Autodesk Inventor part; units mm, degrees
ref_plane "YZ Plane" through (0, 0, 0) normal (1, 0, 0) x (0, 1, 0)
ref_plane "XZ Plane" through (0, 0, 0) normal (0, 1, 0) x (-1, 0, 0)
ref_plane "XY Plane" through (0, 0, 0) normal (0, 0, 1) x (1, 0, 0)
sketch "Sketch1" plane through (0, 0, 0) normal (0, 0, 1) x (1, 0, 0)
  line L0 (0, 0) -> (20, 0)
  line L1 (20, 0) -> (20, 20)
  line L2 (15, 25) -> (5, 25)
  line L3 (0, 20) -> (0, 0)
  circle A0 centre (5, 12.5) radius 1.6
  circle A1 centre (15, 12.5) radius 1.6
  line L4 (5, 25) -> (0, 20)
  line L5 (15, 25) -> (20, 20)
  line L6 (2.1625, 0) -> (2.1625, -6.35)
  line L7 (2.1625, -6.35) -> (5.3375, -6.35)
  line L8 (5.3375, -6.35) -> (5.3375, 0)
  line L9 (14.6625, 0) -> (14.6625, -6.35)
  line L10 (14.6625, -6.35) -> (17.8375, -6.35)
  line L11 (17.8375, -6.35) -> (17.8375, 0)
  point P0 (20, 25)
  point P1 (0, 25)
  dimension "d0" = 25
  dimension "d1" = 20
  dimension "d2" = 3.2
  dimension "d3" = 5
  dimension "d4" = 12.5
  dimension "d7" = 5
  dimension "d8" = 12.5
  dimension "d9" = 5
  dimension "d10" = 5
  dimension "d11" = 5
  dimension "d12" = 5
  dimension "d13" = 3.175
  dimension "d14" = 6.35
  dimension "d15" = 9.325
  dimension "d16" = 2.1625
  dimension "d17" = 2.1625
extrude "Extrusion1" add sketch "Sketch1" along normal blind 3.175
sketch "Sketch2" plane through (14.6625, -6.35, 0) normal (0, -1, 0) x (1, 0, 0)
  line L0 (0, 0) -> (3.175, 0)
  line L1 (3.175, 0) -> (3.175, 3.175)
  line L2 (0, 3.175) -> (3.175, 3.175)
  line L3 (0, 0) -> (0, 3.175)
  circle A0 centre (1.5875, 1.5875) radius 1.5875
  point P0 (-14.6625, 0)
extrude "Extrusion2" cut sketch "Sketch2" against normal blind 6.35 contours L3 A0 L0 | A0 L1 L0 | L3 L2 A0 | A0 L2 L1
sketch "Sketch3" plane through (2.1625, -6.35, 0) normal (0, -1, 0) x (1, 0, 0)
  line L0 (0, 0) -> (3.175, 0)
  line L1 (3.175, 0) -> (3.175, 3.175)
  line L2 (0, 3.175) -> (3.175, 3.175)
  line L3 (0, 0) -> (0, 3.175)
  circle A0 centre (1.5875, 1.5875) radius 1.5875
  point P0 (-2.1625, 0)
extrude "Extrusion3" cut sketch "Sketch3" against normal blind 6.35 contours L3 A0 L0 | A0 L1 L0 | L3 L2 A0 | A0 L2 L1
equation "\"d7\" = d3"
equation "\"d8\" = d4"
equation "\"d16\" = d17"
properties part number "Effector_ZProbe_A"
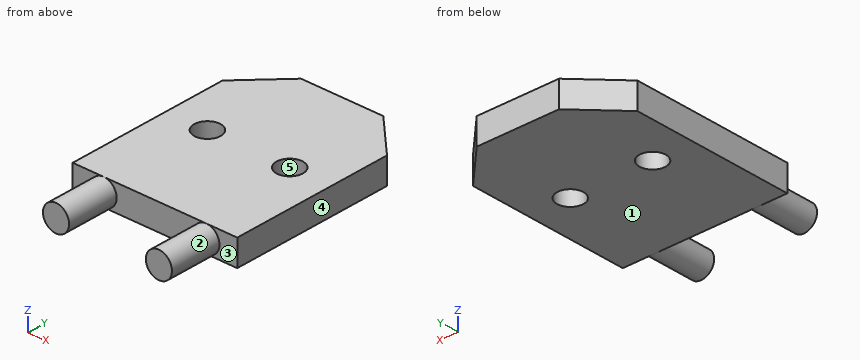
Input: part model. Units: mm. Frame: model coordinates. Face numbers are marked on the shaded views. A direction names the side the tool comes from. Give positions to 0.01 mm unless a question says otherwise; leave off trailing zeros. Loops run counter-clockwise (first coordinate to the right, second up) from the corner with the lowest first, then second, coordinate; pieces in that order, holes last.
1) Mould query, pull axis Y, two halves, no side actions, for the marked faces 3, 4 and 5. Classes: released by +Y, released by -Y, zero draft, split by the parting line, or undercut.
A:
face 3: released by -Y
face 4: zero draft
face 5: undercut
2) Contact query for flat-ended pins moving along their axis: pin 1 (1 mm diameter, centred on x = 9.5, z = 1, fed in from -Y); pin 2 (1 mm diameter, centred on x = 18, z = 1, fed in from -Y). Output: stop coordinate, or through.
A:
pin 1: stops at y = 0
pin 2: stops at y = -6.35
3) Section query B-B on z = 1.25. Return the cut outline in (x, y), and give its area (3 significant figures).
A:
outline: (0, 0) - (2.2, 0) - (2.2, -6.35) - (5.3, -6.35) - (5.3, 0) - (14.7, 0) - (14.7, -6.35) - (17.8, -6.35) - (17.8, 0) - (20, 0) - (20, 20) - (15, 25) - (5, 25) - (0, 20) - close; hole circle Ø3.2 at (5, 12.5); hole circle Ø3.2 at (15, 12.5)
area: 498 mm2
4) Section query D-D on x = 2.5. Return the cut outline in (y, z) (3 decimals), and give its area (3 significant figures).
A:
outline: (-6.35, 0.609) - (0, 0.609) - (0, 0) - (22.5, 0) - (22.5, 3.175) - (0, 3.175) - (0, 2.566) - (-6.35, 2.566) - close
area: 83.9 mm2
5) Reachability of the marked faces 1 and 2 from +Z, -Z, +X, -X, +Y, -Y: full face, straight path, thin tool, end or side. Return the list, or none.
A:
face 1: -Z, +X, -X, +Y, -Y
face 2: -Y
6) Line query: L1, parallel to Y at x = 15, z = 2.4; L2, parallel to X at y = 13.5, z = 1.7; L3, parallel to Y at x = 4.5, z = 1.5. Output: solid intervals per line, ascending.
A:
L1: y = -6.35 to 10.9, 14.1 to 25
L2: x = 0 to 3.75, 6.25 to 13.75, 16.25 to 20
L3: y = -6.35 to 10.98, 14.02 to 24.5
7) Section query A-A on y = 12.5. Return the cut outline in (x, z) (3 decimals), and give its area (3 significant figures).
A:
outline: (0, 0) - (3.4, 0) - (3.4, 3.175) - (0, 3.175) - close; (6.6, 0) - (13.4, 0) - (13.4, 3.175) - (6.6, 3.175) - close; (16.6, 0) - (20, 0) - (20, 3.175) - (16.6, 3.175) - close
area: 43.2 mm2
8) Section query C-C on x = 4.5. Return the cut outline in (y, z) (3 decimals).
A:
outline: (-6.35, 0.188) - (0, 0.188) - (0, 0) - (10.98, 0) - (10.98, 3.175) - (0, 3.175) - (0, 2.987) - (-6.35, 2.987) - close; (14.02, 0) - (24.5, 0) - (24.5, 3.175) - (14.02, 3.175) - close
